from build123d import *

# Parameters (mm, degrees)
SKETCH1_R             = 58
BOSS_EXTRUDE1_DEPTH   = 38.1
SKETCH2_R             = 48
CUT_EXTRUDE1_DEPTH    = 28.1
SKETCH5_R             = 2.6
FASTENING_HOLES_DEPTH = 91.441196365
SKETCH9_R             = 36.2
CUT_EXTRUDE2_DEPTH    = 9
SKETCH10_R            = 30
CUT_EXTRUDE3_DEPTH    = 88.033384399
SKETCH6_R             = 2.2
CUT_EXTRUDE4_DEPTH    = 91.441196365
SKETCH16_R            = 3.7
CUT_EXTRUDE5_DEPTH    = 2.2


with BuildPart() as part:
    # Sketch1 → Boss-Extrude1 (new body)
    with BuildSketch(Plane(origin=(0, 0, 0), x_dir=(1, 0, 0), z_dir=(0, 1, 0))):
        with Locations(Location((0, 0, 0), (0, 0, 90))):
            Circle(SKETCH1_R)
    extrude(amount=BOSS_EXTRUDE1_DEPTH)

    # Sketch2 → Cut-Extrude1 (cut)
    with BuildSketch(Plane(origin=(0, 38.1, 0), x_dir=(1, 0, 0), z_dir=(0, 1, 0))):
        with Locations(Location((0, 0, 0), (0, 0, 270))):
            Circle(SKETCH2_R)
    extrude(amount=-CUT_EXTRUDE1_DEPTH, mode=Mode.SUBTRACT)

    # Sketch5 → Fastening Holes (cut, through all)
    with BuildSketch(Plane(origin=(0, 38.1, 0), x_dir=(1, 0, 0), z_dir=(0, 1, 0))):
        with Locations(Location((0, 52.731846387, 0), (0, 0, 270))):
            Circle(SKETCH5_R)
        with Locations(Location((33.895377494, 40.3949379, 0), (0, 0, 270))):
            Circle(SKETCH5_R)
        with Locations(Location((51.930731153, 9.15678903, 0), (0, 0, 270))):
            Circle(SKETCH5_R)
        with Locations(Location((45.66711856, -26.365923194, 0), (0, 0, 270))):
            Circle(SKETCH5_R)
        with Locations(Location((18.035353659, -49.55172693, 0), (0, 0, 270))):
            Circle(SKETCH5_R)
        with Locations(Location((-18.035353659, -49.55172693, 0), (0, 0, 270))):
            Circle(SKETCH5_R)
        with Locations(Location((-45.66711856, -26.365923194, 0), (0, 0, 270))):
            Circle(SKETCH5_R)
        with Locations(Location((-51.930731153, 9.15678903, 0), (0, 0, 270))):
            Circle(SKETCH5_R)
        with Locations(Location((-33.895377493, 40.3949379, 0), (0, 0, 270))):
            Circle(SKETCH5_R)
    extrude(amount=-FASTENING_HOLES_DEPTH, mode=Mode.SUBTRACT)

    # Sketch9 → Cut-Extrude2 (cut)
    with BuildSketch(Plane.XZ):
        with Locations(Location((0, 0, 0), (0, 0, 270))):
            Circle(SKETCH9_R)
    extrude(amount=-CUT_EXTRUDE2_DEPTH, mode=Mode.SUBTRACT)

    # Sketch10 → Cut-Extrude3 (cut, through all)
    with BuildSketch(Plane.XZ.offset(-9)):
        with Locations(Location((0, 0, 0), (0, 0, 270))):
            Circle(SKETCH10_R)
    extrude(amount=-CUT_EXTRUDE3_DEPTH, mode=Mode.SUBTRACT)

    # Sketch6 → Cut-Extrude4 (cut, through all)
    with BuildSketch(Plane.XZ):
        with Locations(Location((13.13322, -40.419902677, 0), (0, 0, 270))):
            Circle(SKETCH6_R)
        with Locations(Location((-13.133224522, -40.419901208, 0), (0, 0, 270))):
            Circle(SKETCH6_R)
        with Locations(Location((-34.383223658, -24.980871299, 0), (0, 0, 270))):
            Circle(SKETCH6_R)
        with Locations(Location((-42.5, 2.377e-06, 0), (0, 0, 270))):
            Circle(SKETCH6_R)
        with Locations(Location((-34.383220864, 24.980875146, 0), (0, 0, 270))):
            Circle(SKETCH6_R)
        with Locations(Location((-13.13322, 40.419902677, 0), (0, 0, 270))):
            Circle(SKETCH6_R)
        with Locations(Location((13.133224522, 40.419901208, 0), (0, 0, 270))):
            Circle(SKETCH6_R)
        with Locations(Location((34.383223658, 24.980871299, 0), (0, 0, 270))):
            Circle(SKETCH6_R)
        with Locations(Location((42.5, -2.377e-06, 0), (0, 0, 270))):
            Circle(SKETCH6_R)
        with Locations(Location((34.383220864, -24.980875146, 0), (0, 0, 270))):
            Circle(SKETCH6_R)
    extrude(amount=-CUT_EXTRUDE4_DEPTH, mode=Mode.SUBTRACT)

    # Sketch16 → Cut-Extrude5 (cut)
    with BuildSketch(Plane.XZ):
        with Locations(Location((-13.13322, 40.419902677, 0), (0, 0, 270))):
            Circle(SKETCH16_R)
        with Locations(Location((13.133224522, 40.419901208, 0), (0, 0, 270))):
            Circle(SKETCH16_R)
        with Locations(Location((34.383223658, 24.980871299, 0), (0, 0, 270))):
            Circle(SKETCH16_R)
        with Locations(Location((42.5, -2.377e-06, 0), (0, 0, 270))):
            Circle(SKETCH16_R)
        with Locations(Location((34.383220864, -24.980875146, 0), (0, 0, 270))):
            Circle(SKETCH16_R)
        with Locations(Location((13.13322, -40.419902677, 0), (0, 0, 270))):
            Circle(SKETCH16_R)
        with Locations(Location((-13.133224522, -40.419901208, 0), (0, 0, 270))):
            Circle(SKETCH16_R)
        with Locations(Location((-34.383223658, -24.980871299, 0), (0, 0, 270))):
            Circle(SKETCH16_R)
        with Locations(Location((-42.5, 2.377e-06, 0), (0, 0, 270))):
            Circle(SKETCH16_R)
        with Locations(Location((-34.383220864, 24.980875146, 0), (0, 0, 270))):
            Circle(SKETCH16_R)
    extrude(amount=-CUT_EXTRUDE5_DEPTH, mode=Mode.SUBTRACT)


solid = part.part
For this review, take the finished solid that the model builds, in its own axes (mm). A direction names the side the tool comes from. Coordinates: 2 decimals unless noted, no trailing zeros. Loops run counter-clockwise (first coordinate to the right, second up) from the corner with the lowest first, then second, coordinate; pieces in that order, holes last. Notation, with made-up numbers: (-15, 7) - (27, 7) arc R24 cw to (27, 30) - close; hole circle Ø2 at (-32.5, -30). An arc over 180 degrees is marked (long way). Return JSON: item names as keys, results as strings.
Item 1: Take a section at A-A (z = 0). State how many separate pieces and enclosed holes the cut face has, then the cut area to 3 significant figures.
Determined:
{"separate pieces": "4", "enclosed holes": "0", "area": "909 mm2"}
Item 2: Take a section at B-B (x = 0). Give the boundary of the cut face in (y, z).
Determined:
{"outline": "(0, -58) - (38.1, -58) - (38.1, -55.33) - (0, -55.33) - close; (0, -50.13) - (38.1, -50.13) - (38.1, -48) - (10, -48) - (10, -30) - (9, -30) - (9, -36.2) - (0, -36.2) - close; (0, 36.2) - (9, 36.2) - (9, 30) - (10, 30) - (10, 48) - (38.1, 48) - (38.1, 58) - (0, 58) - close"}
Item 3: For faces 4 (the flat face through (33, 2.2, -27)), 5 (the cylindrical face through (-14, 6, 38.4)), list the 3-axis set-ups (+Z, -Z, +X, -X, +Y, -Y) from which the entire face can be reached by the end or side of a thin tool; tool diameter is ignored.
Determined:
{"face 4": "-Y", "face 5": "+Y, -Y"}
Item 4: Insertion check: pin 1 (3 mm diameter, centred on x = 24, y = 29.5, fed in from -Z); pin 2 (1 mm diameter, centred on x = 5, z = 29, fed in from +Y); pin 3 (12 mm diameter, centred on x = 34.5, y = 14, fed in from -Z); pin 4 (5 mm diameter, centred on x = 31, z = -9.5, fed in from +Y). Each pin has a flat end and moves straight along its axis. Give the tip position at first contact, or say it passes through.
Determined:
{"pin 1": "stops at z = -53.46", "pin 2": "passes through", "pin 3": "stops at z = -50.51", "pin 4": "stops at y = 10"}
Item 5: Take a section at C-C (z = 15). Give the boundary of the cut face in (x, y), then the cut area to 3 significant figures.
Determined:
{"outline": "(-56.03, 0) - (-32.95, 0) - (-32.95, 9) - (-25.98, 9) - (-25.98, 10) - (-45.6, 10) - (-45.6, 38.1) - (-56.03, 38.1) - close; (25.98, 9) - (32.95, 9) - (32.95, 0) - (56.03, 0) - (56.03, 38.1) - (45.6, 38.1) - (45.6, 10) - (25.98, 10) - close", "area": "1,060 mm2"}
Item 6: For line 1 (X direction, y = 6, z = 0); line 2 (X direction, y = 9.6, z = 0); line 3 (Z direction, x = 32, y = 19), list the stretches that pass through material, from the lowest coordinate up.
Determined:
{"line 1": "x = -58 to -44.7, -40.3 to -36.2, 36.2 to 40.3, 44.7 to 58", "line 2": "x = -58 to -44.7, -40.3 to -30, 30 to 40.3, 44.7 to 58", "line 3": "z = -48.37 to -42.17, -38.62 to -35.78, 35.78 to 48.37"}
Item 7: Mouldability with a two-part tool opening along Z and no side actions: class faces 1 (the cylindrical face through (33.54, 6.05, 22.95)), 2 (the cylindrical face through (22.21, 18.78, -53.58)), 3 (the flat face through (21.21, 38.1, 43.23)) as pulls with the +Z half, pulls with the -Z half, needs draft (parallel to the pull), parting line crosses it, or undercut.
Determined:
{"face 1": "undercut", "face 2": "parting line crosses it", "face 3": "needs draft"}
